Could you check a few things on this model? Use its own coordinates, in mm. A direction names the side the tool comes from. Give positions to 0.01 mm unless a question says otherwise; leave off trailing zeros. Order: outer loops, then holes, each group sorted by start corner. A loop starts at its lowest first (then second) coordinate and runs counter-clockwise, first axis right, second up. Notation, with made-up numbers: M -11,88.5 L 18,88.5 A24 cw 18,104.5 Z; hole C 29.25,-35.75 d1. An arc over 180 degrees is marked long. Return JSON: item names as keys, results as strings. Group by question number.
```python
from build123d import *

# Parameters (mm, degrees)
SKETCH1_W           = 100.584
SKETCH1_H           = 26.67
SKETCH1_R           = 3.302
BOSS_EXTRUDE1_DEPTH = 2.54
SKETCH2_W           = 64.516
SKETCH2_H           = 26.67
BOSS_EXTRUDE2_DEPTH = 49.53
CUT_EXTRUDE1_REACH  = 28.67
FILLET1_R           = 25.4


with BuildPart() as part:
    # Sketch1 → Boss-Extrude1 (new body)
    with BuildSketch(Plane.XY):
        with Locations((-0.466217893, 3.598360719)):
            Rectangle(SKETCH1_W, SKETCH1_H)
        with Locations((-41.106217893, 9.059360719)):
            Circle(SKETCH1_R, mode=Mode.SUBTRACT)
        with Locations((40.173782107, 9.059360719)):
            Circle(SKETCH1_R, mode=Mode.SUBTRACT)
    extrude(amount=BOSS_EXTRUDE1_DEPTH)

    # Sketch2 → Boss-Extrude2 (add)
    with BuildSketch(Plane.XY.offset(2.54)):
        with Locations((-0.466217893, 3.598360719)):
            Rectangle(SKETCH2_W, SKETCH2_H)
    extrude(amount=BOSS_EXTRUDE2_DEPTH)

    # Sketch5 → Cut-Extrude1 (cut, up to next)
    with BuildSketch(Plane.XZ.offset(9.736639281), mode=Mode.PRIVATE) as cut_extrude1_sk1:
        with BuildLine():
            ThreePointArc((24.933782107, 22.86), (-1.101416548, 48.252056291), (-25.834448025, 21.59))
            Line((-25.834448025, 21.59), (24.902012238, 21.59))
            ThreePointArc((24.902012238, 21.59), (24.925838398, 22.224801345), (24.933782107, 22.86))
        make_face()
    cut_extrude1_tool1 = extrude(cut_extrude1_sk1.sketch, amount=-CUT_EXTRUDE1_REACH, mode=Mode.PRIVATE) & part.part
    add(cut_extrude1_tool1.solids().sort_by_distance((-0.466218, -9.736639, 32.957158))[0], mode=Mode.SUBTRACT)
    # Sketch5 → Cut-Extrude1 (cut, up to next)
    with BuildSketch(Plane.XZ.offset(9.736639281), mode=Mode.PRIVATE) as cut_extrude1_sk2:
        with BuildLine():
            ThreePointArc((-25.834448025, 21.59), (-21.643974867, 8.836355339), (-11.53782121, 0))
            Line((-11.53782121, 0), (10.605385423, 0))
            ThreePointArc((10.605385423, 0), (20.71153908, 8.836355339), (24.902012238, 21.59))
            Line((24.902012238, 21.59), (-25.834448025, 21.59))
        make_face()
    cut_extrude1_tool2 = extrude(cut_extrude1_sk2.sketch, amount=-CUT_EXTRUDE1_REACH, mode=Mode.PRIVATE) & part.part
    add(cut_extrude1_tool2.solids().sort_by_distance((-0.466218, -9.736639, 11.906571))[0], mode=Mode.SUBTRACT)
    # Sketch5 → Cut-Extrude1 (cut, up to next)
    with BuildSketch(Plane.XZ.offset(9.736639281), mode=Mode.PRIVATE) as cut_extrude1_sk3:
        with BuildLine():
            Line((-30.946217893, 21.59), (-30.946217893, 0))
            Line((-30.946217893, 0), (-11.53782121, 0))
            ThreePointArc((-11.53782121, 0), (-21.643974867, 8.836355339), (-25.834448025, 21.59))
            Line((-25.834448025, 21.59), (-30.946217893, 21.59))
        make_face()
    cut_extrude1_tool3 = extrude(cut_extrude1_sk3.sketch, amount=-CUT_EXTRUDE1_REACH, mode=Mode.PRIVATE) & part.part
    add(cut_extrude1_tool3.solids().sort_by_distance((-25.424083, -9.736639, 8.295091))[0], mode=Mode.SUBTRACT)
    # Sketch5 → Cut-Extrude1 (cut, up to next)
    with BuildSketch(Plane.XZ.offset(9.736639281), mode=Mode.PRIVATE) as cut_extrude1_sk4:
        with BuildLine():
            ThreePointArc((24.902012238, 21.59), (20.71153908, 8.836355339), (10.605385423, 0))
            Line((10.605385423, 0), (30.013782107, 0))
            Line((30.013782107, 0), (30.013782107, 21.59))
            Line((30.013782107, 21.59), (24.902012238, 21.59))
        make_face()
    cut_extrude1_tool4 = extrude(cut_extrude1_sk4.sketch, amount=-CUT_EXTRUDE1_REACH, mode=Mode.PRIVATE) & part.part
    add(cut_extrude1_tool4.solids().sort_by_distance((24.491648, -9.736639, 8.295091))[0], mode=Mode.SUBTRACT)

    # Fillet1
    fillet1_edges = [part.edges().sort_by_distance(p)[0] for p in [
        (-32.724217893, 3.598360719, 52.07),
        (31.791782107, 3.598360719, 52.07),
    ]]
    fillet(fillet1_edges, radius=FILLET1_R)


solid = part.part
```
1. For pin 1 (10 mm diameter, centred on y = 5.5, z = 30, fed in from -X); pin 2 (1 mm diameter, centred on y = 8.5, z = 29.5, fed in from -X); pin 3 (10.5 mm diameter, centred on x = -41.11, y = 9.06, fed in from +Z), each with a flat end and sliding along its axis, tell me the tip position at first contact or that it passes through.
2. If we mould it in two halves opening along X, with no side actions, what happens to faces 4 (the flat face through (49.826, 3, 1)), 5 (the flat face through (-30.946, 3, 11)), 6 (the flat face through (-42, 4, 2.54))? For each: pulls with the +X half, pulls with the -X half, needs draft (parallel to the pull), parting line crosses it, or undercut.
3. Imagine slicing it at C-C, the plane x = -16. Please give me the cut outline in (y, z), plus the area to 3 significant figures.
4. Which directions (+Z, -Z, +X, -X, +Y, -Y) give clear straight access to the entire face, cutting with the end or side of a thin tool? Please do faces 1 (the flat face through (-1, 4, 52.07)), 2 (the flat face through (30.014, 3, 11)), 3 (the flat face through (41, 4, 2.54)).
5. I need wall thicknesses on L1, parallel to X at y = 10, z = 10.5; L2, parallel to X at y = 15, z = 31; L3, parallel to Z at x = -39, y = 13.25. Which ranges of each line are inside material? Lowest first, please. Write a range as from..to.
6. Imagine slicing it at A-A, the plane z = 12. Please give me the cut outline in (x, y).
7. Imagine slicing it at B-B, the plane x = 33. Please give me the cut outline in (y, z).
Values:
{
 "1": {"pin 1": "stops at x = -32.72", "pin 2": "stops at x = -32.62", "pin 3": "stops at z = 2.54"},
 "2": {"face 4": "pulls with the +X half", "face 5": "undercut", "face 6": "needs draft"},
 "3": {"outline": "M -9.74,42.96 L 16.93,42.96 L 16.93,50.54 L -9.74,50.54 Z", "area": "202 mm²"},
 "4": {"face 1": "+Z, +X, -X, +Y, -Y", "face 2": "-Z, +Y, -Y", "face 3": "+Z, +X, +Y, -Y"},
 "5": {"L1": "x = -32.72..-30.95, 30.01..31.79", "L2": "x = -32.35..-24.53, 23.59..31.42", "L3": "z = 0..2.54"},
 "6": {"outline": "M -32.72,-9.74 L -30.95,-9.74 L -30.95,16.93 L -32.72,16.93 Z; M 30.01,-9.74 L 31.79,-9.74 L 31.79,16.93 L 30.01,16.93 Z"},
 "7": {"outline": "M -9.74,0 L 16.93,0 L 16.93,2.54 L -9.74,2.54 Z"}
}
